Design review of the part built by this model. Coordinates are the model's own, in mm. Face numbers are marked on the shaded views. A direction names the side the tool comes from. Give positions to 0.01 mm unless a question says otherwise; leave off trailing zeros. Loops run counter-clockwise (first coordinate to the right, second up) from the corner with the lowest first, then second, coordinate; pieces in that order, holes last. Notation, with made-up numbers: (46, 43.5) - (87, 43.5) arc R19 cw to (87, 67.5) - close; hole circle Ø7 at (49, 68). An arc over 180 degrees is marked (long way). Put each result on its own line as item: value. Start each with the question number.
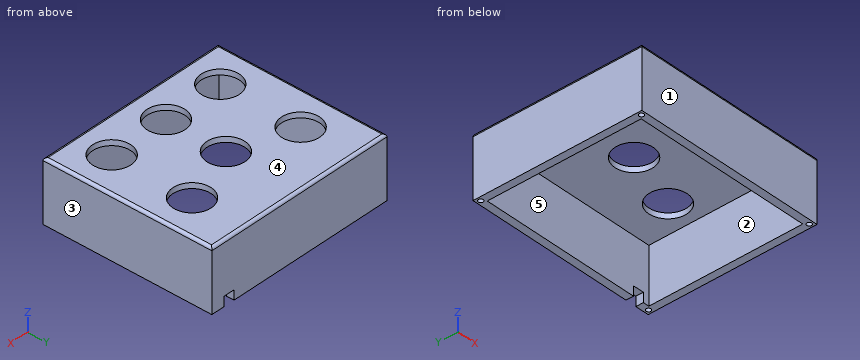
```python
from build123d import *

# Parameters (mm, degrees)
SKETCH_W        = 142
SKETCH_H        = 124
SKETCH_R        = 14
PAD_DEPTH       = 45
SKETCH001_W     = 131
SKETCH001_H     = 113
POCKET_DEPTH    = 41
SKETCH002_R     = 1.75
POCKET001_DEPTH = 6
SKETCH003_W     = 8
SKETCH003_H     = 7
POCKET002_DEPTH = 10
FILLET_R        = 2


with BuildPart() as part:
    # Sketch → Pad (new body)
    with BuildSketch(Plane.XY):
        Rectangle(SKETCH_W, SKETCH_H)
        with Locations((0, 8)):
            Circle(SKETCH_R, mode=Mode.SUBTRACT)
        with Locations((0, -36)):
            Circle(SKETCH_R, mode=Mode.SUBTRACT)
        with Locations((44, -36)):
            Circle(SKETCH_R, mode=Mode.SUBTRACT)
        with Locations((-44, -36)):
            Circle(SKETCH_R, mode=Mode.SUBTRACT)
        with Locations((-44, 23)):
            Circle(SKETCH_R, mode=Mode.SUBTRACT)
        with Locations((44, 23)):
            Circle(SKETCH_R, mode=Mode.SUBTRACT)
    extrude(amount=PAD_DEPTH)

    # Sketch001 (on Face11 of Pad) → Pocket (cut)
    with BuildSketch(Plane(origin=(0, 0, 0), x_dir=(1, 0, 0), z_dir=(0, 0, -1))):
        Rectangle(SKETCH001_W, SKETCH001_H)
    extrude(amount=-POCKET_DEPTH, mode=Mode.SUBTRACT)

    # Sketch002 (on Face4 of Pocket) → Pocket001 (cut)
    with BuildSketch(Plane(origin=(0, 0, 0), x_dir=(1, 0, 0), z_dir=(0, 0, -1))):
        with Locations((-68, 59)):
            Circle(SKETCH002_R)
        with Locations((-68, -59)):
            Circle(SKETCH002_R)
        with Locations((68, -59)):
            Circle(SKETCH002_R)
        with Locations((68, 59)):
            Circle(SKETCH002_R)
    extrude(amount=-POCKET001_DEPTH, mode=Mode.SUBTRACT)

    # Sketch003 (on Face2 of Pocket001) → Pocket002 (cut)
    with BuildSketch(Plane(origin=(0, 62, 0), x_dir=(-1, 0, 0), z_dir=(0, 1, 0))):
        with Locations((-57, 3.5)):
            Rectangle(SKETCH003_W, SKETCH003_H)
    extrude(amount=-POCKET002_DEPTH, mode=Mode.SUBTRACT)

    # Fillet
    fillet_edges = [part.edges().sort_by_distance(p)[0] for p in [
        (-71, 0, 45),
        (0, 62, 45),
        (71, 0, 45),
        (0, -62, 45),
    ]]
    fillet(fillet_edges, radius=FILLET_R)


solid = part.part
```
Item 1: Consider section A-A (x = -27). State the section outline as (y, z) points.
Item 2: For L1, parallel to Y at x = -44, z = 43.3; L2, parallel to Y at x = -68, z = 1.35; L3, parallel to X at y = 59, z = 2, list the stretches that pass through material, from the lowest coordinate up. Write a range as from..to.
Item 3: Machinability: for the marked faces 1 and 2, which of the approach directions +Z, -Z, +X, -X, +Y, -Y give a long, thin tool a straight path to every point of the face, cutting with its end or side? Answer none if there is none.
Item 4: Mouldability with a two-part tool opening along X and no side actions: class the marked faces 3, 4 and 5 as pulls with the +X half, pulls with the -X half, needs draft (parallel to the pull), parting line crosses it, or undercut.
Item 5: Consider section C-C (x = 44). State the section outline as (y, z) points.
Item 6: Consider section D-D (y = 49). State the section outline as (x, z) points.
Item 7: For P1, Ø6, axis at x = 55.5, y = 59, coming from the -Z side; P2, Ø4, axis at x = 0, y = -16.5, coming from the -Z side; P3, Ø22.5, axis at x = -44, y = -36, coming from the +Z side, all flat-tipped, find the tip position at first contact; note any pin that passes through.
Item 8: Consider section B-B (z = 23). State the section outline as (x, y) points.
Geometry says:
1. outline: (-62, 0) - (-56.5, 0) - (-56.5, 41) - (56.5, 41) - (56.5, 0) - (62, 0) - (62, 43) arc R2 ccw to (60, 45) - (-60, 45) arc R2 ccw to (-62, 43) - close
2. L1: y = -61.98..-50, -22..9, 37..61.98
2. L2: y = -62..-60.75, -57.25..57.25, 60.75..62
2. L3: x = -71..-69.75, -66.25..53, 61..66.25, 69.75..71
3. face 1: +Z, -Z, +X, -X, -Y
3. face 2: -Z
4. face 3: pulls with the +X half
4. face 4: needs draft
4. face 5: undercut
5. outline: (-62, 0) - (-56.5, 0) - (-56.5, 41) - (-50, 41) - (-50, 45) - (-60, 45) arc R2 ccw to (-62, 43) - close; (-22, 41) - (9, 41) - (9, 45) - (-22, 45) - close; (37, 41) - (56.5, 41) - (56.5, 0) - (62, 0) - (62, 43) arc R2 ccw to (60, 45) - (37, 45) - close
6. outline: (-71, 0) - (-65.5, 0) - (-65.5, 41) - (65.5, 41) - (65.5, 0) - (71, 0) - (71, 43) arc R2 ccw to (69, 45) - (-69, 45) arc R2 ccw to (-71, 43) - close
7. P1: stops at z = 0
7. P2: stops at z = 41
7. P3: passes through
8. outline: (-71, -62) - (71, -62) - (71, 62) - (-71, 62) - close; hole (-65.5, -56.5) - (65.5, -56.5) - (65.5, 56.5) - (-65.5, 56.5) - close
